Build history of the part. All positions in model axes, mm. A direction names the side the tool comes from. Round coordinates to 2 decimals unless told otherwise and drop trailing zeros. Write each loop counter-clockwise with the first axis right and the second up, starting at its lowest first coordinate (ties: lowest second). Pieces come first, ordered by that corner, then holes. Notation, with made-up numbers: M 12.5,-25.75 L 58.5,-25.75 A14 cw 58.5,-6.75 Z; hole C 46,46.25 d4. An arc over 180 degrees is marked long. Write item = value, one per line. Start each with the question number.
Q1. Band-saw the part on C-C on x = -8.5. Write the cut outline in (y, z), plus the area to 3 significant figures.
Q2. Pull direction X, two halves, no side cores. Call faces 1 (the flat face through (29.25, 2, 13)), 2 (the cylindrical face through (15.15, 6.64, 25.59)), 3 (the flat face through (0, -1.5, 26)), 4 (the flat face through (-28, 7.5, 13)): released by +X, released by -X, zero draft, split by the parting line, or undercut.
Q3. Band-saw the part on A-A on y = 2.5. Write the cut outline in (x, z), plus the area to 3 significant figures.
Q4. Tool access for faces 5 (the cylindrical face through (-26.22, -6, 13.36)), 6 (the flat face through (0, -9.1, 13)), 7 (the flat face through (14.25, 3, 1)): list every direction of +Z, -Z, +X, -X, +Y, -Y with a clear straight run to the whole face (end or side of a thin tool).
Q5. Drop flat-ended pins along their axis: P1, Ø6, axis at y = -6.5, z = 14, coming from the +X side; P2, Ø6, axis at y = -6.5, z = 13, coming from the -X side; P3, Ø1.5, axis at y = -4.5, z = 3.5, coming from the -X side. Give the stop position or say it passes through.
Q6. Band-saw the part on D-D on y = -6.5. Write the cut outline in (x, z).
Q7. Probe L1, parallel to Z at x = 9.5, y = -7.25; L2, parallel to X at y = 2.5, z = 3.25; L3, parallel to X at y = 1.5, z = 25. List the from-to ranges inside material, lowest first.
Q8. Band-saw the part on B-B on z = 10. Write the cut outline in (x, y), plus the area to 3 significant figures.
```python
from build123d import *

# Parameters (mm, degrees)
F1_DEPTH = 26.4
F2_R     = 6.6
F3_T     = -1.6
F4_W     = 28.5
F4_H     = 9
F5_DEPTH = 26.401
F6_R     = 3


with BuildPart() as f1:
    # F0 (on Top) → F1 (new body)
    with BuildSketch(Plane.XY):
        Polygon((29.25, 7.5), (27.65, 7.5), (-27.65, 7.5), (-29.25, 7.5), (-29.25, -9.1), (29.25, -9.1), align=None)
    extrude(amount=F1_DEPTH)

    # F2
    f2_edges = [f1.edges().sort_by_distance(p)[0] for p in [
        (29.25, -9.1, 13.2),
        (-29.25, -9.1, 13.2),
    ]]
    fillet(f2_edges, radius=F2_R)

    # F3
    f3_openings = [f1.faces().sort_by_distance(p)[0] for p in [
        (0, 7.5, 13.2),
    ]]
    offset(amount=F3_T, openings=f3_openings)

    # F4 (on face) → F5 (cut, through all)
    with BuildSketch(Plane.XY.offset(26.4)):
        with Locations((0, 3)):
            Rectangle(F4_W, F4_H)
    extrude(amount=-F5_DEPTH, mode=Mode.SUBTRACT)

    # F6
    f6_edges = [f1.edges().sort_by_distance(p)[0] for p in [
        (14.25, -1.5, 25.6),
        (14.25, 7.5, 25.6),
        (14.25, 7.5, 0.8),
        (14.25, -1.5, 0.8),
        (-14.25, 7.5, 25.6),
        (-14.25, 7.5, 0.8),
        (-14.25, -1.5, 0.8),
        (-14.25, -1.5, 25.6),
    ]]
    fillet(f6_edges, radius=F6_R)


solid = f1.part
```
Conclusion:
q1.outline = M -9.1,0 L -1.5,0 L -1.5,1.6 L -7.5,1.6 L -7.5,24.8 L -1.5,24.8 L -1.5,26.4 L -9.1,26.4 Z
q1.area = 61.4 mm^2
q2.face_1 = released by +X
q2.face_2 = undercut
q2.face_3 = undercut
q2.face_4 = zero draft
q3.outline = M -29.25,0 L -14.25,0 L -14.25,1.6 L -27.65,1.6 L -27.65,24.8 L -14.25,24.8 L -14.25,26.4 L -29.25,26.4 Z; M 14.25,0 L 29.25,0 L 29.25,26.4 L 14.25,26.4 L 14.25,24.8 L 27.65,24.8 L 27.65,1.6 L 14.25,1.6 Z
q3.area = 170 mm^2
q4.face_5 = +Y
q4.face_6 = +Z, -Z, +X, -X, -Y
q4.face_7 = +Z, -Z, +Y
q5.P1 = 29.17
q5.P2 = -29.17
q5.P3 = -29.13
q6.outline = M -27.9,0 L 27.9,0 L 27.9,26.4 L -27.9,26.4 Z; hole M -25.65,1.6 L 25.65,1.6 L 25.65,24.8 L -25.65,24.8 Z
q7.L1 = 0 to 1.6, 24.8 to 26.4
q7.L2 = -29.25 to -27.65, 27.65 to 29.25
q7.L3 = -29.25 to -14.25, 14.25 to 29.25
q8.outline = M -29.25,-2.5 A6.6 ccw -22.65,-9.1 L 22.65,-9.1 A6.6 ccw 29.25,-2.5 L 29.25,7.5 L 27.65,7.5 L 27.65,-2.5 A5 cw 22.65,-7.5 L -22.65,-7.5 A5 cw -27.65,-2.5 L -27.65,7.5 L -29.25,7.5 Z
q8.area = 134 mm^2
